```python
from build123d import *

# Parameters (mm, degrees)
SKETCH1_W           = 320
SKETCH1_H           = 80
SKETCH1_W_2         = 5
SKETCH1_H_2         = 50
BOSS_EXTRUDE1_DEPTH = 10
SKETCH2_W           = 320
SKETCH2_H           = 20
BOSS_EXTRUDE2_DEPTH = 10
SKETCH3_R           = 1.5
CUT_EXTRUDE1_DEPTH  = 10


with BuildPart() as part:
    # Sketch1 → Boss-Extrude1 (new body)
    with BuildSketch(Plane(origin=(0, 0, 0), x_dir=(1, 0, 0), z_dir=(0, 1, 0))):
        with Locations((160, -40)):
            Rectangle(SKETCH1_W, SKETCH1_H)
        with Locations((12.5, -40)):
            Rectangle(SKETCH1_W_2, SKETCH1_H_2, mode=Mode.SUBTRACT)
        with Locations((59.5, -40)):
            Rectangle(SKETCH1_W_2, SKETCH1_H_2, mode=Mode.SUBTRACT)
        with Locations((307.5, -40)):
            Rectangle(SKETCH1_W_2, SKETCH1_H_2, mode=Mode.SUBTRACT)
    extrude(amount=BOSS_EXTRUDE1_DEPTH)

    # Sketch2 → Boss-Extrude2 (add)
    with BuildSketch(Plane(origin=(0, 10, 0), x_dir=(1, 0, 0), z_dir=(0, 1, 0))):
        with Locations((160, 10)):
            Rectangle(SKETCH2_W, SKETCH2_H)
        with Locations((160, -90)):
            Rectangle(SKETCH2_W, SKETCH2_H)
    extrude(amount=-BOSS_EXTRUDE2_DEPTH)

    # Sketch3 → Cut-Extrude1 (cut)
    with BuildSketch(Plane(origin=(0, 10, 0), x_dir=(1, 0, 0), z_dir=(0, 1, 0))):
        with Locations(Location((152, 15, 0), (0, 0, 270))):
            Circle(SKETCH3_R)
        with Locations(Location((152, -95, 0), (0, 0, 90))):
            Circle(SKETCH3_R)
    extrude(amount=-CUT_EXTRUDE1_DEPTH, mode=Mode.SUBTRACT)


solid = part.part
```
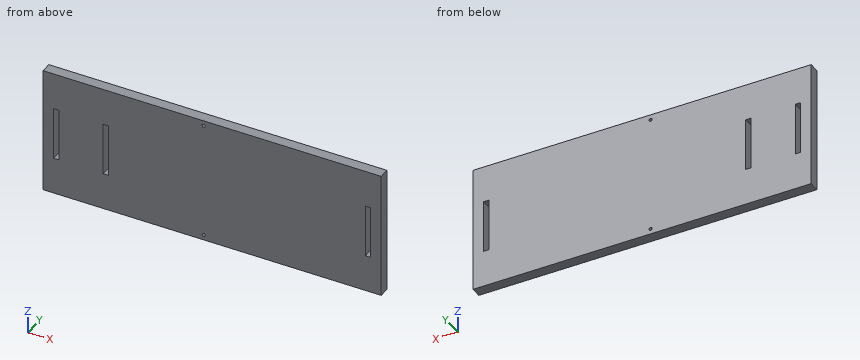
Can you work these out from the model? Positions are in its coordinate system, mm. Coordinates: 2 decimals unless noted, no trailing zeros. Loops run counter-clockwise (first coordinate to the right, second up) from the corner with the lowest first, then second, coordinate; pieces in that order, holes last. Notation, with made-up numbers: (73, 86.25) - (116, 86.25) arc R17 cw to (116, 91.25) - close; hole circle Ø8 at (49.5, 48.5). An arc over 180 degrees is marked (long way). Use a Markdown table: item, result.
Item 1: I want a section at B-B on z = 44. Please give me the cut outline in (x, y).
Numbers:
| item | result |
|---|---|
| outline | (0, 0) - (10, 0) - (10, 10) - (0, 10) - close; (15, 0) - (57, 0) - (57, 10) - (15, 10) - close; (62, 0) - (305, 0) - (305, 10) - (62, 10) - close; (310, 0) - (320, 0) - (320, 10) - (310, 10) - close |
Item 2: If I drill on probe 1 along Z at (x, y) = (152, 6.75); probe 2 along X at (y, z) = (7.5, 25); probe 3 along X at (y, z) = (3.5, -15), over which ranges is the centre line in solid material (lowest first)? Write a range as from..to.
Numbers:
| item | result |
|---|---|
| probe 1 | z = -20..-16.5, -13.5..93.5, 96.5..100 |
| probe 2 | x = 0..10, 15..57, 62..305, 310..320 |
| probe 3 | x = 0..150.5, 153.5..320 |
Item 3: Will this pin go through, and if not, where does the flat tip stop? pin 1 (2.5 mm diameter, centred on x = 152, z = 95, fed in from +Y).
Numbers:
| item | result |
|---|---|
| pin 1 | passes through |
Item 4: I want a section at A-A on y = 7.25. Please give me the cut outline in (x, z).
Numbers:
| item | result |
|---|---|
| outline | (0, -20) - (320, -20) - (320, 100) - (0, 100) - close; hole (10, 15) - (15, 15) - (15, 65) - (10, 65) - close; hole (57, 15) - (62, 15) - (62, 65) - (57, 65) - close; hole circle Ø3 at (152, -15); hole circle Ø3 at (152, 95); hole (305, 15) - (310, 15) - (310, 65) - (305, 65) - close |
